Model file for the job. Use its own axes, mm. Face numbers are marked on the shaded views. A direction names the side the tool comes from. Give positions to 0.01 mm unless a question says otherwise; leave off trailing zeros. Write each loop counter-clockwise with the first axis right and the second up, starting at its lowest first coordinate (ties: lowest second). Pieces come first, ordered by that corner, then holes.
```python
from build123d import *

# Parameters (mm, degrees)
SKETCH271_R     = 4
PAD109_DEPTH    = 10
SKETCH272_R     = 4
SKETCH272_R_2   = 2.1
PAD110_DEPTH    = 2
SKETCH273_R     = 1.5
POCKET132_DEPTH = 4.001


with BuildPart() as part:
    # Sketch271 → Pad109 (new body)
    with BuildSketch(Plane.XY):
        Circle(SKETCH271_R)
        with BuildLine():
            Line((-1.360147, 1.6), (1.360147, 1.6))
            ThreePointArc((-1.360147, 1.6), (0, -2.1), (1.360147, 1.6))
        make_face(mode=Mode.SUBTRACT)
    extrude(amount=PAD109_DEPTH)

    # Sketch272 (on Face5 of Pad109) → Pad110 (join)
    with BuildSketch(Plane.XY.offset(10)):
        Circle(SKETCH272_R)
        Circle(SKETCH272_R_2, mode=Mode.SUBTRACT)
    extrude(amount=PAD110_DEPTH)

    # Sketch273 → Pocket132 (cut, through all)
    with BuildSketch(Plane.XZ):
        with Locations((0, 8.5)):
            Circle(SKETCH273_R)
    extrude(amount=-POCKET132_DEPTH, mode=Mode.SUBTRACT)


with BuildPart() as part_1:
    # Body097 placement: moved
    add(part.part.moved(Location((0, 11, 0))))


solid = part_1.part
```
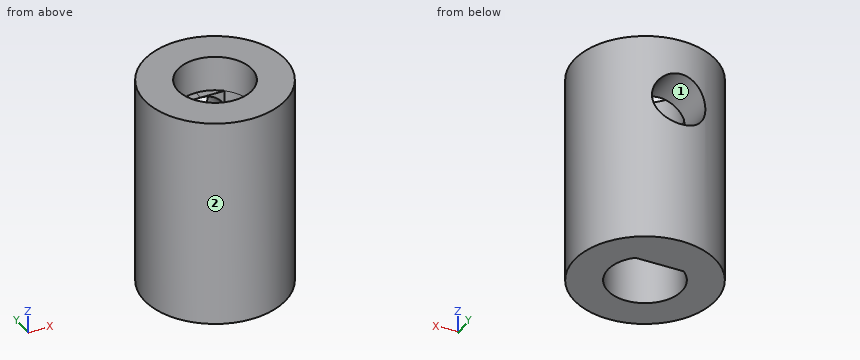
1. Probe probe 1 along Z at (x, y) = (0, 14.4); probe 2 along Y at (x, z) = (0, 11.6); probe 3 along X at (y, z) = (13.2, 8.5). List the from-to ranges inside material, lowest first.
Calculated:
probe 1: z = 0 to 7, 10 to 12
probe 2: y = 7 to 8.9, 13.1 to 15
probe 3: x = -3.34 to -1.5, 1.5 to 3.34
2. Which spindle directions (+Z, -Z, +X, -X, +Y, -Y) get a long thin tool onto all of the face, cutting with end or side? Do the marked faces 1 and 2. Say none if no direction does.
Calculated:
face 1: +Y
face 2: +Z, -Z
3. Slice it at C-C, the plane x = -0.5. Write the cut outline in (y, z), and give its area (3 significant figures).
Calculated:
outline: (7.03, 0) - (8.96, 0) - (8.96, 12) - (7.03, 12) - close; (12.6, 0) - (14.97, 0) - (14.97, 7.09) - (12.6, 7.09) - close; (12.6, 9.91) - (14.97, 9.91) - (14.97, 12) - (13.04, 12) - (13.04, 10) - (12.6, 10) - close
area: 44.0 mm2
4. Pin check, flat tips, straight feed: P1, Ø2.5, axis at x = 0, y = 11, coming from the -Z side; P2, Ø1, axis at x = -1, z = 9.5, coming from the -Y side; P3, Ø1.5, axis at y = 8.5, z = 8, coming from the -X side. Stop position of each tip, or through.
Calculated:
P1: passes through
P2: stops at y = 7.03
P3: stops at x = -3.6
5. Slice it at D-D, the plane z = 10.75. Write the cut outline in (x, y), and give its area (3 significant figures).
Calculated:
outline: circle Ø8 at (0, 11); hole circle Ø4.2 at (0, 11)
area: 36.4 mm2
6. Slice it at B-B, the plane x = 1.75. Write the cut outline in (y, z), and give its area (3 significant figures).
Calculated:
outline: (7.4, 0) - (9.84, 0) - (9.84, 12) - (7.4, 12) - close; (12.16, 0) - (14.6, 0) - (14.6, 12) - (12.16, 12) - close
area: 58.5 mm2
7. Slice it at A-A, the plane y = 11. Write the cut outline in (x, z), and give its area (3 significant figures).
Calculated:
outline: (-4, 0) - (-2.1, 0) - (-2.1, 12) - (-4, 12) - close; (2.1, 0) - (4, 0) - (4, 12) - (2.1, 12) - close
area: 45.6 mm2
